from build123d import *

# Parameters (mm, degrees)
BOSS_EXTRUDE1_DEPTH = 20
BOSS_EXTRUDE2_START = 20
SKETCH1_3_R         = 10
BOSS_EXTRUDE2_DEPTH = 50
SKETCH2_R           = 15
CUT_EXTRUDE1_DEPTH  = 20
SKETCH3_R           = 21.409884381
BOSS_EXTRUDE3_DEPTH = 15.5
FILLET1_R           = 1.8
FILLET2_R           = 4
FILLET3_R           = 2


with BuildPart() as part:
    # Sketch1 → Boss-Extrude1 (new body)
    with BuildSketch(Plane.XY):
        with BuildLine():
            Line((-75, -335.522292415), (75, -335.522292415))
            Line((75, -335.522292415), (75, -85.522292415))
            ThreePointArc((75, -85.522292415), (108.166019919, -35.201912374), (110.9687456, 25))
            Line((110.9687456, 25), (-110.9687456, 25))
            ThreePointArc((-110.9687456, 25), (-108.166019919, -35.201912374), (-75, -85.522292415))
            Line((-75, -85.522292415), (-75, -335.522292415))
        make_face()
    extrude(amount=BOSS_EXTRUDE1_DEPTH)

    # Sketch1<3> → Boss-Extrude2 (add)
    with BuildSketch(Plane.XY.offset(BOSS_EXTRUDE2_START)):
        Circle(SKETCH1_3_R)
    extrude(amount=BOSS_EXTRUDE2_DEPTH)

    # Sketch2 → Cut-Extrude1 (cut)
    with BuildSketch(Plane.XY.offset(20)):
        with Locations((0, -300)):
            Circle(SKETCH2_R)
    extrude(amount=-CUT_EXTRUDE1_DEPTH, mode=Mode.SUBTRACT)

    # Sketch3 → Boss-Extrude3 (add)
    with BuildSketch(Plane.XY.offset(20)):
        Circle(SKETCH3_R)
    extrude(amount=BOSS_EXTRUDE3_DEPTH)

    # Fillet1
    fillet1_edges = [part.edges().sort_by_distance(p)[0] for p in [
        (-10, 0, 35.5),
    ]]
    fillet(fillet1_edges, radius=FILLET1_R)

    # Fillet2
    fillet2_edges = [part.edges().sort_by_distance(p)[0] for p in [
        (-21.409884381, 0, 20),
    ]]
    fillet(fillet2_edges, radius=FILLET2_R)

    # Fillet3
    fillet3_edges = [part.edges().sort_by_distance(p)[0] for p in [
        (-21.409884381, 0, 35.5),
    ]]
    fillet(fillet3_edges, radius=FILLET3_R)


solid = part.part
Read the model definition and answer for the solid it produces. Units are mm, in the model's axes. A direction names the side the tool comes from. Round coordinates to 2 decimals unless told otherwise and drop trailing zeros. Order: outer loops, then holes, each group sorted by start corner. A loop starts at its lowest first (then second) coordinate and runs counter-clockwise, first axis right, second up.
1) The part is cut by section A-A on y = -300. Write down the section's boundary in (x, z), plus the area to 3 significant figures.
2) Flat-ended cylindrical pins translate along their axes: pin 1 (5 mm diameter, centred on y = -62, z = 17.5, fed in from -X); pin 2 (16 mm diameter, centred on y = -246, z = 8, fed in from +X); pin 3 (2 mm diameter, centred on x = 49, y = -268, fed in from +Z). Find the tip coordinate at first contact, or state that the pin passes through.
3) The part is cut by section B-B on z = 10. Write down the section's boundary in (x, y), plus the area to 3 significant figures.
4) The part is cut by section C-C on y = 0. Write down the section's boundary in (x, z).
5) The part is cut by section D-D on x = -29. Write down the section's boundary in (y, z).
6) Straight lines are drawn through the part: L1, parallel to Y at x = 0, z = 5.25; L2, parallel to Z at x = -44, y = -113.5; L3, parallel to X at y = -273.5, z = 8.5. For each, find the intervals that lie inside material, in ascending order.
7) For faces 1 (the face through (-2.17, -9.76, 53.42)), 2 (the face through (2, 25, 10)), 3 (the face through (-75, -209, 10)), 4 (the face through (75, -212, 10)), determine the directions among +Z, -Z, +X, -X, +Y, -Y from which every point of the face is accessible in a straight line to the end or side of a thin tool.
8) The mould has two halves that part along Y. Classify faces 5 (the face through (-1.953, -285.128, 10.14)), 6 (the face through (0, 0, 70)), 7 (the face through (107.9, -36.01, 9.86)): released by +Y, released by -Y, zero draft, split by the parting line, or undercut.
Resolved:
1. outline: (-75, 0) - (-15, 0) - (-15, 20) - (-75, 20) - close; (15, 0) - (75, 0) - (75, 20) - (15, 20) - close
1. area: 2,400 mm2
2. pin 1: stops at x = -96.95
2. pin 2: stops at x = 75
2. pin 3: stops at z = 20
3. outline: (-110.97, 25) arc R113.75 ccw to (-75, -85.52) - (-75, -335.52) - (75, -335.52) - (75, -85.52) arc R113.75 ccw to (110.97, 25) - close; hole circle Ø30 at (0, -300)
3. area: 59,900 mm2
4. outline: (-113.75, 0) - (113.75, 0) - (113.75, 20) - (25.41, 20) arc R4 cw to (21.41, 24) - (21.41, 33.5) arc R2 ccw to (19.41, 35.5) - (11.8, 35.5) arc R1.8 cw to (10, 37.3) - (10, 70) - (-10, 70) - (-10, 37.3) arc R1.8 cw to (-11.8, 35.5) - (-19.41, 35.5) arc R2 ccw to (-21.41, 33.5) - (-21.41, 24) arc R4 cw to (-25.41, 20) - (-113.75, 20) - close
5. outline: (-335.52, 0) - (25, 0) - (25, 20) - (-335.52, 20) - close
6. L1: y = -335.52 to -315, -285 to 25
6. L2: z = 0 to 20
6. L3: x = -75 to 75
7. face 1: +Z
7. face 2: +Z, -Z, +X, -X, +Y
7. face 3: +Z, -Z, -X, -Y
7. face 4: +Z, -Z, +X, -Y
8. face 5: undercut
8. face 6: zero draft
8. face 7: split by the parting line
